from build123d import *

# Parameters (mm, degrees)
TAPPED_HOLE_FOR_9_16_12_HELICOIL1_D = 14.68374


with BuildPart() as part:
    # Sketch1 → Revolve2 (revolve)
    with BuildSketch(Plane(origin=(0, 0, 0), x_dir=(1, 0, 0), z_dir=(0, 1, 0))):
        Polygon((882.163023054, 111.99614411), (882.163023054, 90.365625069), (901.213023054, 90.365625069), (901.213023054, 109.051426841), align=None)
    revolve(axis=Axis((1002.111866296, 0, -90.365625069), (-1, 0, 0)))

    # Tapped Hole for 9/16-12 Helicoil1 (through all)
    with Locations(Plane.ZY.offset(-882.163023054)):
        with Locations((-90.365625069, 0)):
            Hole(TAPPED_HOLE_FOR_9_16_12_HELICOIL1_D / 2)

    # Sketch5 → Cut-Revolve1 (revolve, cut)
    with BuildSketch(Plane(origin=(0, 0, 0), x_dir=(1, 0, 0), z_dir=(0, 1, 0))):
        with BuildLine():
            Line((928.636701013, 102.242153557), (928.636701013, 100.247495069))
            Line((928.636701013, 100.247495069), (895.498023054, 100.247495069))
            ThreePointArc((895.498023054, 100.247495069), (897.743087084, 101.177431039), (898.673023054, 103.422495069))
            Line((898.673023054, 103.422495069), (898.673023054, 104.151966666))
            ThreePointArc((898.673023054, 104.151966666), (897.908477535, 106.21844536), (895.983048759, 107.289700731))
            Line((895.983048759, 107.289700731), (928.636701013, 102.242153557))
        make_face()
    revolve(axis=Axis((1002.111866296, 0, -90.365625069), (-1, 0, 0)), mode=Mode.SUBTRACT)


solid = part.part
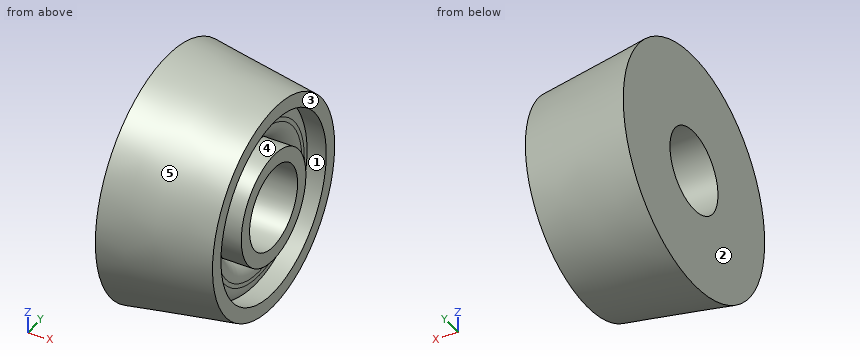
Read the model definition and answer for the solid it produces. Units are mm, in the model's axes. Face numbers are marked on the shaded views. A direction names the side the tool comes from. Give positions to 0.01 mm unless a question says otherwise; leave off trailing zeros. Loops run counter-clockwise (first coordinate to the right, second up) from the corner with the lowest first, then second, coordinate; pieces in that order, holes last. Notation, with made-up numbers: (-5.5, 83) - (21.5, 83) arc R8 cw to (21.5, 97) - close; hole circle Ø5 at (-32.5, 13.5). An arc over 180 degrees is marked (long way). Answer as CSV lines item,"result". Start each with the question number.
1) Straight lines are drawn through the part: L1, parallel to Z at x = 897.75, y = -8; L2, parallel to Z at x = 897.5, y = -11.5; L3, parallel to Z at x = 886.5, y = 3.5. For each, find the intervals that lie inside material, in ascending order. Write a range as from..to.
2) Find section B-B (x = 893.25). Write down the section's boundary in (y, z).
3) Determine the mould class of the marked faces 3, 4 and 5 for opening direction Z: released by +Z, released by -Z, zero draft, split by the parting line, or undercut.
4) Each of these flat-tipped pins is pushed along its axis until it touches: pin 1 Ø5 at (y, z) = (-14.5, -74) entering from -X; pin 2 Ø1 at (x, y) = (888, -2) entering from -Z; pin 3 Ø1 at (x, z) = (895, -100.5) entering from +Y; pin 4 Ø2 at (x, y) = (885.5, -1) entering from +Z. Where does it stop, or does it pass through?
5) Which of the six approach directions +Z, -Z, +X, -X, +Y, -Y give full straight-line access (tool end or side, diameter ignored) to the marked faces 1 and 2?
Findings below:
1,L1,"-107.84..-104.97, -104.25..-97.65, -96.17..-84.56, -83.08..-76.48, -75.76..-72.89"
1,L2,"-105.82..-102.46, -101.85..-78.88, -78.27..-74.92"
1,L3,"-111.03..-96.82, -83.91..-69.7"
2,outline,"circle Ø39.83 at (0, -90.37); hole circle Ø14.68 at (0, -90.37)"
3,face 3,"zero draft"
3,face 4,"undercut"
3,face 5,"split by the parting line"
4,pin 1,"x = 882.16"
4,pin 2,"z = -111.09"
4,pin 3,"y = 17.14"
4,pin 4,"z = -69.11"
5,face 1,"none"
5,face 2,"+Z, -Z, -X, +Y, -Y"
